Part model, mm, in its own coordinate system. A direction names the side the tool comes from. Round coordinates to 2 decimals unless told otherwise and drop trailing zeros. Write each loop counter-clockwise with the first axis right and the second up, starting at its lowest first coordinate (ties: lowest second). Pieces come first, ordered by that corner, then holes. Notation, with made-up numbers: (41, 5.25) -> (85, 5.25) arc R18 cw to (85, 14.25) -> close; hole circle Ø9 at (-25, 24.25). An arc over 180 degrees is marked (long way). Return JSON: item names as keys, results as strings. Group by question number.
(1) Mould opens along Z. For faces 1 (the conical face through (-0.95, 54.51, 33.58)), 2 (the flat face through (2, 74.7, 29.7)), 3 (the flat face through (-47, 145.5, 20)), 4 (the flat face through (-3, 124, 26.5)) say: +Z half, -Z half, draft (parallel to the pull), parting line (faces both ways), or undercut.
(2) Saw through at D-D (x = -20.5). List the corners of the cut face in (y, z).
(3) Saw through at C-C (x = -46). List the corners of the cut face in (y, z).
(4) Drill centre lines: L1, parallel to X at y = 128.5, z = 12; L2, parallel to X at y = 86, z = 2; L3, parallel to Y at x = -46, z = 2.1. Where is each one in solid material? Low to high. Write a range as from..to.
(5) Saw through at B-B (z = 22.5). List the corners of the cut face in (x, y).
(6) Drop flat-ended pins along their axis: pin 1 Ø3 at (x, y) = (-5, 103.5) entering from +Z; pin 2 Ø2 at (y, z) = (147, 31.5) entering from +X; pin 3 Ø4 at (x, z) = (-1.5, 32) entering from -Y. Give the stop position or say it passes through.
(7) Saw through at A-A (y = 86.65). List the corners of the cut face in (x, z).
(8) Tool access for faces 5 (the flat face through (-1, 74, 13)), 6 (the flat face through (-4, 25, 26.5)), 7 (the flat face through (-5.5, 74, 16)): list every direction of +Z, -Z, +X, -X, +Y, -Y with a clear straight run to the whole face (end or side of a thin tool).
from build123d import *

# Parameters (mm, degrees)
SKETCH010_W     = 90
SKETCH010_H     = 150
PAD004_DEPTH    = 35
SKETCH011_W     = 81
SKETCH011_H     = 141
POCKET004_DEPTH = 30.5
SKETCH012_R     = 5.5
PAD005_DEPTH    = 150
SKETCH015_W     = 50.5
SKETCH015_H     = 14
POCKET006_DEPTH = 7.5
PAD007_DEPTH    = 49
SKETCH024_R     = 39
POCKET009_DEPTH = 5


with BuildPart() as part:
    # Sketch010 → Pad004 (new body)
    with BuildSketch(Plane.XY):
        with Locations((-46, 75)):
            Rectangle(SKETCH010_W, SKETCH010_H)
    extrude(amount=PAD004_DEPTH)

    # Sketch011 (on Face6 of Pad004) → Pocket004 (cut)
    with BuildSketch(Plane.XY.offset(35)):
        with Locations((-46, 75)):
            Rectangle(SKETCH011_W, SKETCH011_H)
    extrude(amount=-POCKET004_DEPTH, mode=Mode.SUBTRACT)

    # Sketch012 → Pad005 (join)
    with BuildSketch(Plane.XZ):
        with Locations((-0.5, 35)):
            Circle(SKETCH012_R)
    extrude(amount=-PAD005_DEPTH)

    # Sketch015 → Pocket006 (cut, symmetric)
    with BuildSketch(Plane.YZ):
        with Locations((25.25, 33.5)):
            Rectangle(SKETCH015_W, SKETCH015_H)
        with Locations((124.75, 33.5)):
            Rectangle(SKETCH015_W, SKETCH015_H)
    extrude(amount=POCKET006_DEPTH, both=True, mode=Mode.SUBTRACT)

    # Sketch016 (on Face13 of Pocket006) → Pad007 (join)
    with BuildSketch(Plane.XZ.offset(-50.5)):
        Polygon((-1, 26.7), (5, 32.7), (5, 35), (-1, 35), align=None)
    extrude(amount=-PAD007_DEPTH)

    # Sketch020 (on DatumPlane) → Groove (revolve, cut)
    with BuildSketch(Plane(origin=(-0.5, 99.5, 0), x_dir=(0, -1, 0), z_dir=(-1, 0, 0))):
        Polygon((-1, 28.5), (5.5, 35), (-1, 35), align=None)
        Polygon((50, 28.5), (43.5, 35), (50, 35), align=None)
    revolve(axis=Axis((-0.5, 94, 35), (0, 1, 0)), mode=Mode.SUBTRACT)

    # Sketch024 (on Face18 of Groove) → Pocket009 (cut)
    with BuildSketch(Plane.XY.offset(4.5)):
        with Locations((-46, 86.65)):
            Circle(SKETCH024_R)
    extrude(amount=-POCKET009_DEPTH, mode=Mode.SUBTRACT)


solid = part.part
Computed values:
{
 "1": {"face 1": "undercut", "face 2": "-Z half", "face 3": "draft", "face 4": "+Z half"},
 "2": {"outline": "(0, 0) -> (57.14, 0) -> (57.14, 4.5) -> (4.5, 4.5) -> (4.5, 35) -> (0, 35) -> close; (116.16, 0) -> (150, 0) -> (150, 35) -> (145.5, 35) -> (145.5, 4.5) -> (116.16, 4.5) -> close"},
 "3": {"outline": "(0, 0) -> (47.65, 0) -> (47.65, 4.5) -> (4.5, 4.5) -> (4.5, 35) -> (0, 35) -> close; (125.65, 0) -> (150, 0) -> (150, 35) -> (145.5, 35) -> (145.5, 4.5) -> (125.65, 4.5) -> close"},
 "4": {"L1": "-91..-86.5, -5.5..-1", "L2": "-91..-84.99, -7.01..-1", "L3": "0..47.65, 125.65..150"},
 "5": {"outline": "(-91, 0) -> (-1, 0) -> (-1, 150) -> (-91, 150) -> close; hole (-86.5, 4.5) -> (-5.5, 4.5) -> (-5.5, 145.5) -> (-86.5, 145.5) -> close"},
 "6": {"pin 1": "z = 26.5", "pin 2": "x = -7.5", "pin 3": "y = 50.84"},
 "7": {"outline": "(-91, 0) -> (-85, 0) -> (-85, 4.5) -> (-86.5, 4.5) -> (-86.5, 35) -> (-91, 35) -> close; (-7, 0) -> (-1, 0) -> (-1, 26.7) -> (5, 32.7) -> (5, 35) arc R5.5 ccw (long way) to (-5.5, 32.71) -> (-5.5, 4.5) -> (-7, 4.5) -> close"},
 "8": {"face 5": "-Z, +X, +Y, -Y", "face 6": "+Z, +X, -Y", "face 7": "none"}
}
